```python
from build123d import *

# Parameters (mm, degrees)
F0_R        = 3
F1_DEPTH    = 5
F2_T1_DEPTH = 32.3482938807
F3_R        = 5


# Not quite as in the source:
# - a fillet or chamfer that OpenCascade refuses, or shapes differently, is made with other operations: its cross-section is extruded or revolved along the edge and cut away or added


with BuildPart() as f1:
    # F0 (on Front) → F1 (new body)
    with BuildSketch(Plane.XZ):
        Polygon((0, 30), (0, 0), (10, 0), (10, 10), (15.5, 10), (15.5, 0), (165.5, 0), (165.5, 20), (148, 50.3108891325), (143.6698729811, 47.8108891325), (161.1698729811, 17.5), (158.1387840678, 15.75), (128.1387840678, 67.7115242271), align=None)
        with Locations((123.1387840678, 60)):
            Circle(F0_R, mode=Mode.SUBTRACT)
        Polygon((165.5, 20), (165.5, 0), (225.5, 0), (225.5, 10), (148, 50.3108891325), align=None)
    extrude(amount=F1_DEPTH)

    # F2: fillet of radius 10 on 1 edges, made by hand

    # F2_s2 → F2_t1 (cut)
    with BuildSketch(Plane.XZ.offset(-13.6741469404)):
        with BuildLine():
            ThreePointArc((152.8524940595, 47.7869104222), (148.2640985796, 48.9152185915), (143.6698729811, 47.8108891325))
            Line((143.6698729811, 47.8108891325), (148, 50.3108891325))
            Line((148, 50.3108891325), (152.8524940595, 47.7869104222))
        make_face()
    extrude(amount=F2_T1_DEPTH, mode=Mode.SUBTRACT)

    # F3
    f3_edges = [f1.edges().sort_by_distance(p)[0] for p in [
        (225.5, -2.5, 10),
        (0, -2.5, 30),
    ]]
    fillet(f3_edges, radius=F3_R)


solid = f1.part
```
Here's how the part is built. I have some questions about the finished solid (model axes, mm). A direction names the side the tool comes from. Round coordinates to 2 decimals unless told otherwise and drop trailing zeros. Loops run counter-clockwise (first coordinate to the right, second up) from the corner with the lowest first, then second, coordinate; pieces in that order, holes last. Notation, with made-up numbers: (-33, 43) -> (-14, 43) arc R20 ccw to (-14, 60) -> close; hole circle Ø7 at (61.5, 65.5). An arc over 180 degrees is marked (long way). Answer as CSV lines item,"result". Start each with the question number.
1. Imagine slicing it at C-C on x = 138.5. Write out the boundary of the cut face in (y, z).
2. I need wall thicknesses on probe 1 along X at (y, z) = (-3.2, 5); probe 2 along Z at (x, y) = (155.5, -3.2); probe 3 along X at (y, z) = (-2.6, 16.5). Which ranges of each line are inside material? Lowest first, please. Write a range as from..to.
3. If we mould it in two halves opening along Z, with no side actions, what happens to faces 1 (the face through (119, -2, 0)), 2 (the face through (143.349, -2.465, 41.367)), 3 (the face through (0, -2, 13))? For each: pulls with the +Z half, pulls with the -Z half, needs draft (parallel to the pull), parting line crosses it, or undercut.
4. Imagine slicing it at A-A on z = 60. Write out the boundary of the cut face in (x, y), plus the area to 3 significant figures.
5. I'm going to push flat-ended pins straight in: P1, Ø1.5, axis at x = 12.5, y = -3, coming from the -Z side; P2, Ø3, axis at y = -4.5, z = 47.5, coming from the +X side. Where does each tip first touch, or does it pass through?
6. Imagine slicing it at D-D on z = 51. Write out the boundary of the cut face in (x, y).
7. For faces 4 (the face through (10, -2, 5)), 5 (the face through (111, -5, 27)), 6 (the face through (152.297, -2.465, 32.868)), which set-ups out of +Z, -Z, +X, -X, +Y, -Y let a thin tool reach every point of the face, with its end or its side?
8. Imagine slicing it at B-B on y = -3.1. Write out the boundary of the cut face in (x, z).
Solution:
1,outline,"(-5, 0) -> (0, 0) -> (0, 49.77) -> (-5, 49.77) -> close"
2,probe 1,"0..10, 15.5..225.5"
2,probe 2,"0..20.32, 27.32..46.41"
2,probe 3,"0..157.71, 159.44..213"
3,face 1,"pulls with the -Z half"
3,face 2,"undercut"
3,face 3,"needs draft"
4,outline,"(101.94, -5) -> (120.14, -5) -> (120.14, 0) -> (101.94, 0) -> close; (126.14, -5) -> (132.59, -5) -> (132.59, 0) -> (126.14, 0) -> close"
4,area,"123 mm²"
5,P1,"z = 10"
5,P2,"x = 156.29"
6,outline,"(71.36, -5) -> (137.79, -5) -> (137.79, 0) -> (71.36, 0) -> close"
7,face 4,"-Z, +Y, -Y"
7,face 5,"+Z, -Z, +X, -X, -Y"
7,face 6,"+Y, -Y"
8,outline,"(0, 0) -> (10, 0) -> (10, 10) -> (15.5, 10) -> (15.5, 0) -> (225.5, 0) -> (225.5, 6.96) arc R5 ccw to (222.81, 11.4) -> (152.85, 47.79) arc R10 ccw to (143.67, 47.81) -> (161.17, 17.5) -> (158.14, 15.75) -> (128.14, 67.71) -> (3.59, 31.06) arc R5 ccw to (0, 26.26) -> close; hole circle Ø6 at (123.14, 60)"
